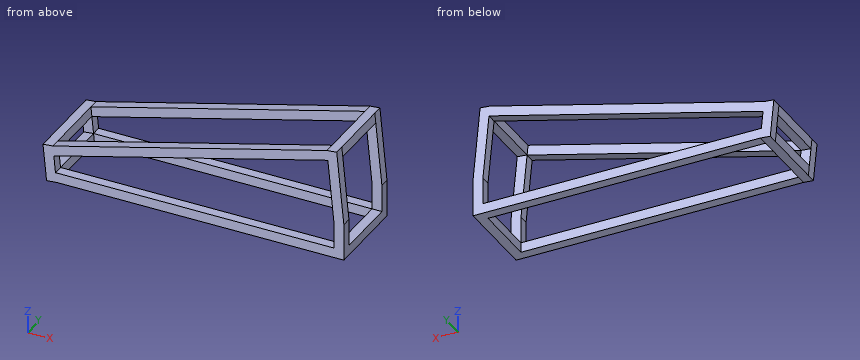
```python
from build123d import *

# Parameters (mm, degrees)
F1_DEPTH = 40
F3_W     = 40
F3_H     = 40
F4_DEPTH = 130


with BuildPart() as f1:
    # F0 (on Front) → F1 (new body)
    with BuildSketch(Plane.XZ):
        Polygon((-1215.873162, 146.164695), (-1201.424196, -3.835305), (-1161.60849, 0), (0, 0), (0, 150), (-28.764789, 448.617794), (-68.580495, 444.782489), (-1176.057456, 150), align=None)
        Polygon((-1172.169917, 109.642031), (-64.692955, 404.42452), (-40, 148.07792), (-40, 40), (-1165.461548, 40), align=None, mode=Mode.SUBTRACT)
    extrude(amount=F1_DEPTH)

    # F3 (on face) → F4 (join)
    with BuildSketch(Plane.XZ):
        Polygon((-24.929484, 408.802088), (-28.764789, 448.617794), (-68.580495, 444.782489), (-64.74519, 404.966783), align=None)
        with Locations((-20, 20)):
            Rectangle(F3_W, F3_H)
        Polygon((-1172.222151, 110.184294), (-1176.057456, 150), (-1215.873162, 146.164695), (-1212.037857, 106.348989), align=None)
        Polygon((-1161.60849, 0), (-1165.443796, 39.815706), (-1205.259501, 35.980401), (-1201.424196, -3.835305), align=None)
    extrude(amount=-F4_DEPTH)

    # F5: F1 across face


with BuildPart() as f1_1:
    add(f1.part)
    add(f1.part.mirror(Plane(origin=(-46.754989, 130, 426.792288), x_dir=(1, 0, 0), z_dir=(0, 1, 0))))


solid = f1_1.part
```
Model file for the job. Use its own axes, mm. Give positions to 0.01 mm unless a question says otherwise; leave off trailing zeros. Loops run counter-clockwise (first coordinate to the right, second up) from the corner with the lowest first, then second, coordinate; pieces in that order, holes last. Notation, with made-up numbers: M 52.5,74.5 L 68.5,74.5 A17 ccw 68.5,88.5 Z; hole C 45,0.5 d4. An arc over 180 degrees is marked long. Use one line per item in the form item = value.
Item 1: Slice it at A-A on y = 102. List the corners of the cut face in (x, z).
Filled in:
outline = M -1215.87,146.16 L -1212.04,106.35 L -1172.22,110.18 L -1176.06,150 Z; M -1205.26,35.98 L -1201.42,-3.84 L -1161.61,0 L -1165.44,39.82 Z; M -68.58,444.78 L -64.75,404.97 L -24.93,408.8 L -28.76,448.62 Z; M -40,0 L 0,0 L 0,40 L -40,40 Z
Item 2: Flat gauge pins, fed straight in: pin 1 Ø12 at (x, y) = (-585.5, 272) entering from +Z; pin 2 Ø20 at (y, z) = (154.5, 26.5) entering from -X; pin 3 Ø3 at (y, z) = (1, 360.5) entering from +X. Where does each tip first touch, or does it go through?
Filled in:
pin_1 = 308.79
pin_2 = -1205.26
pin_3 = -20.17
Item 3: Slice it at B-B on x = -228. List the corners of the cut face in (y, z).
Filled in:
outline = M -40,0 L 0,0 L 0,40 L -40,40 Z; M -40,360.96 L 0,360.96 L 0,402.35 L -40,402.35 Z; M 260,0 L 300,0 L 300,40 L 260,40 Z; M 260,360.96 L 300,360.96 L 300,402.35 L 260,402.35 Z
Item 4: Drill centre lines: L1, parallel to X at y = 249, z = 24.5; L2, parallel to X at y = -15.5, z = 96; L3, parallel to X at y = 24, z = 138. Where is each one in solid material? Low to high.
Filled in:
L1 = -1204.15 to -1163.97, -40 to 0
L2 = -1211.04 to -1170.86, -40 to 0
L3 = -1215.09 to -1174.9
